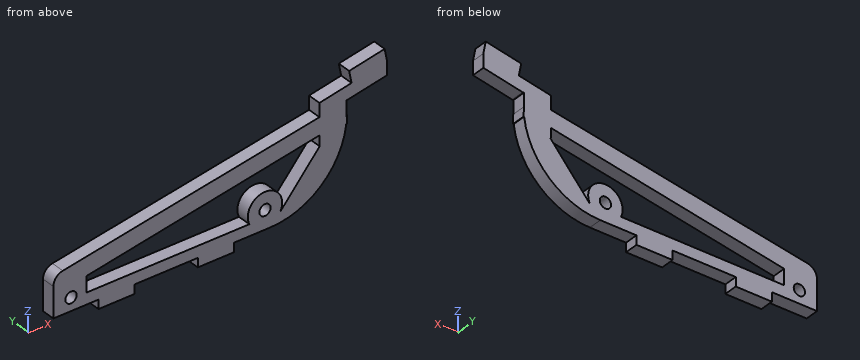
from build123d import *

# Parameters (mm, degrees)
F0_R     = 3.175
F1_DEPTH = 3.81


with BuildPart() as f1:
    # F0 (on Front) → F1 (new body, symmetric)
    with BuildSketch(Plane.XZ):
        with BuildLine():
            Line((-59.890088, -21.828954), (-59.890088, -16.748955))
            Line((-59.890088, -16.748955), (-24.330088, -16.748955))
            Line((-24.330088, -16.748955), (-24.330088, -21.828954))
            Line((-24.330088, -21.828954), (-4.010088, -21.828954))
            Line((-4.010088, -21.828954), (-4.010088, -16.748955))
            Line((-4.010088, -16.748955), (16.322047, -16.748955))
            ThreePointArc((16.322047, -16.748955), (44.998655, -5.847431), (59.191398, 21.351045))
            ThreePointArc((59.191398, 21.351045), (59.276078, 22.127556), (59.346694, 22.905473))
            Line((59.346694, 22.905473), (59.346694, 34.051045))
            Line((59.346694, 34.051045), (60.017541, 34.051045))
            Line((60.017541, 34.051045), (82.11488, 38.268742))
            Line((82.11488, 38.268742), (82.11488, 45.888742))
            Line((82.11488, 45.888742), (80.789338, 52.833516))
            Line((80.789338, 52.833516), (60.82966, 49.023833))
            Line((60.82966, 49.023833), (62.155202, 42.079058))
            Line((62.155202, 42.079058), (44.106369, 38.634096))
            Line((44.106369, 38.634096), (44.106369, 31.014096))
            Line((44.106369, 31.014096), (-100.318861, 6.59136))
            ThreePointArc((-100.318861, 6.59136), (-104.110125, 4.428987), (-105.610088, 0.33025))
            Line((-105.610088, 0.33025), (-105.610088, -16.748954))
            Line((-105.610088, -16.748954), (-80.210088, -16.748954))
            Line((-80.210088, -16.748954), (-80.210088, -21.828954))
            Line((-80.210088, -21.828954), (-59.890088, -21.828954))
        make_face()
        with Locations((-95.69665, -9.482743)):
            Circle(F0_R, mode=Mode.SUBTRACT)
        with BuildLine():
            Line((-87.117024, -1.517896), (44.106369, 21.351045))
            Line((44.106369, 21.351045), (44.224798, 15.474893))
            Line((44.224798, 15.474893), (22.260441, -10.339289))
            ThreePointArc((22.260441, -10.339289), (13.454788, 3.430057), (4.649135, -10.339289))
            Line((4.649135, -10.339289), (-87.117024, -10.339289))
            Line((-87.117024, -10.339289), (-87.117024, -1.517896))
        make_face(mode=Mode.SUBTRACT)
        with Locations((13.454788, -6.276863)):
            Circle(F0_R, mode=Mode.SUBTRACT)
        with BuildLine():
            ThreePointArc((59.346694, 22.905473), (59.276078, 22.127556), (59.191398, 21.351045))
            Line((59.191398, 21.351045), (59.346694, 21.351045))
            Line((59.346694, 21.351045), (59.346694, 22.905473))
        make_face()
        with BuildLine():
            ThreePointArc((59.489912, 26.418909), (59.454092, 24.660732), (59.346694, 22.905473))
            Line((59.346694, 22.905473), (59.346694, 21.351045))
            Line((59.346694, 21.351045), (59.489912, 21.351045))
            Line((59.489912, 21.351045), (59.489912, 26.418909))
        make_face()
    extrude(amount=F1_DEPTH, both=True)


solid = f1.part
The model under review builds one solid part; all positions refer to its coordinate system, in mm. Round coordinates to 2 decimals unless told otherwise and drop trailing zeros. Order: outer loops, then holes, each group sorted by start corner. A loop starts at its lowest first (then second) coordinate and runs counter-clockwise, first axis right, second up. Notation, with made-up numbers: (48.25, -29.5) -> (83.25, -29.5) arc R22 ccw to (83.25, -19.5) -> close; hole circle Ø8 at (1.25, 31). An arc over 180 degrees is marked (long way). Use CSV: the item, a comma, the result in double quotes. Start each with the question number.
(1) Consider section A-A on x = -51. Write out the cut boundary in (y, z), and give its area (3 significant figures).
(2) Insertion check: pin 1 (4 mm diameter, centred on x = -76, y = 1, fed in from +Z); pin 2 (2.5 mm diameter, centred on y = -1.5, z = 31, fed in from +X); pin 3 (2.5 mm diameter, centred on y = 0, z = 24, fed in from +X); pin 4 (4 mm diameter, centred on y = 0, z = -18.5, fed in from -X). Each pin has a flat end and moves straight along its axis. Give the tip position at first contact, or say it passes through.
(3) Consider section C-C on x = 14. Write out the cut boundary in (y, z), and give its area (3 significant figures).
(4) Consider section B-B on y = -2. State how many separate pieces and enclosed holes the cut face has, and give its area (3 significant figures).
(5) Consider section D-D on x = -13. Write out the cut boundary in (y, z).
(6) Wall thickness on probe 1 along X at (y, z) = (3.25, -9.5); probe 2 along Z at (x, y) = (26, 2); probe 3 along Z at (x, y) = (28, -0.5): over which ranges is each line inside the solid? List them lowest first. Write a range as from..to.
Responses:
1,outline,"(-3.81, -16.75) -> (3.81, -16.75) -> (3.81, -10.34) -> (-3.81, -10.34) -> close; (-3.81, 4.78) -> (3.81, 4.78) -> (3.81, 14.93) -> (-3.81, 14.93) -> close"
1,area,"126 mm²"
2,pin 1,"z = 11.04"
2,pin 2,"x = 59.35"
2,pin 3,"x = 59.49"
2,pin 4,"x = -105.61"
3,outline,"(-3.81, -16.75) -> (3.81, -16.75) -> (3.81, -9.4) -> (-3.81, -9.4) -> close; (-3.81, -3.15) -> (3.81, -3.15) -> (3.81, 3.41) -> (-3.81, 3.41) -> close; (-3.81, 16.1) -> (3.81, 16.1) -> (3.81, 25.92) -> (-3.81, 25.92) -> close"
3,area,"181 mm²"
4,separate pieces,"1"
4,enclosed holes,"3"
4,area,"4,030 mm²"
5,outline,"(-3.81, -21.83) -> (3.81, -21.83) -> (3.81, -10.34) -> (-3.81, -10.34) -> close; (-3.81, 11.4) -> (3.81, 11.4) -> (3.81, 21.36) -> (-3.81, 21.36) -> close"
6,probe 1,"-105.61..-98.87, -92.52..-87.12, 4.31..22.6, 22.97..40.27"
6,probe 2,"-15.65..-5.94, 18.2..27.95"
6,probe 3,"-15.14..-3.59, 18.54..28.29"
